Read the model definition and answer for the solid it produces. Units are mm, in the model's axes. Face numbers are marked on the shaded views. A direction names the side the tool comes from. Coordinates: 2 decimals unless noted, no trailing zeros. Write each loop counter-clockwise with the first axis right and the second up, starting at its lowest first coordinate (ties: lowest second). Pieces come first, ordered by that corner, then holes.
(1) Find the intervals of material crossed by probe 1 along X at (y, z) = (3, 22); probe 2 along X at (y, z) = (-8.5, 15.75) (3 decimals); probe 3 along Z at (x, y) = (-3, -8), in increasing order.
(2) Section D-D on z = 12.7 is taken. State how many separate pieces and enclosed holes the cut face has, then the cut area to 3 significant figures.
(3) Which of the six approach directions +Z, -Z, +X, -X, +Y, -Y give full straight-line access (tool end or side, diameter ignored) to the marked faces 4 and 5?
(4) Section A-A on x = -4 is taken. Write down the section's boundary in (y, z) (3 decimals), then the cut area to 3 significant figures.
(5) Given pin 1 (4 mm diameter, centred on x = -4.5, z = 19, fed in from +Y); pin 2 (2 mm diameter, centred on x = -1, y = 17.5, fed in from -Z); pin 3 (6 mm diameter, centred on y = -9.5, z = 9.5, fed in from +X); pin 4 (2.5 mm diameter, centred on x = 6, z = 15, fed in from +Y), each flat-ended and moving along its own axis, determine where each tip first touches the part or whether it passes through.
(6) Section B-B on y = 3 is taken. Write down the section's boundary in (x, z), then the cut area to 3 significant figures.
(7) The mould has two halves that part along Z. Classify the marked faces 1, 2 and 3: +Z half, -Z half, draft (parallel to the pull), parting line (faces both ways), or undercut.
(8) Section C-C on z = 3.75 is taken. Write down the section's boundary in (x, y) (3 decimals).
from build123d import *

# Parameters (mm, degrees)
BOSS_EXTRUDE1_DEPTH = 25.4
SKETCH2_R           = 6.35
CUT_EXTRUDE1_DEPTH  = 8.89
SKETCH3_R           = 3.175
CUT_EXTRUDE2_DEPTH  = 6.35
SKETCH4_W           = 0.635
SKETCH4_H           = 18.796
CUT_EXTRUDE3_DEPTH  = 40.162657148
SKETCH5_R           = 1.905
CUT_EXTRUDE4_DEPTH  = 40.416561089


with BuildPart() as part:
    # Sketch1 → Boss-Extrude1 (new body)
    with BuildSketch(Plane.XY):
        with BuildLine():
            ThreePointArc((-14.355971037, 17.457748951), (-15.128392597, 15.680502137), (-15.3924, 13.760725746))
            Line((-15.3924, 13.760725746), (-15.3924, 0.762))
            Line((-15.3924, 0.762), (-15.3924, -11.938))
            ThreePointArc((-15.3924, -11.938), (-13.309343428, -16.966943428), (-8.2804, -19.05))
            Line((-8.2804, -19.05), (8.2804, -19.05))
            ThreePointArc((8.2804, -19.05), (13.309343428, -16.966943428), (15.3924, -11.938))
            Line((15.3924, -11.938), (15.3924, 0.762))
            Line((15.3924, 0.762), (15.3924, 13.760725746))
            ThreePointArc((15.3924, 13.760725746), (15.128392597, 15.680502137), (14.355971037, 17.457748951))
            ThreePointArc((14.355971037, 17.457748951), (0, 25.527), (-14.355971037, 17.457748951))
        make_face()
        with BuildLine():
            Line((-9.2964, 0.762), (-9.2964, 13.760725746))
            ThreePointArc((-9.2964, 13.760725746), (-9.258684657, 14.034979516), (-9.14833872, 14.288871918))
            ThreePointArc((-9.14833872, 14.288871918), (0, 19.431), (9.14833872, 14.288871918))
            ThreePointArc((9.14833872, 14.288871918), (9.258684657, 14.034979516), (9.2964, 13.760725746))
            Line((9.2964, 13.760725746), (9.2964, 0.762))
            ThreePointArc((9.2964, 0.762), (8.99882049, 0.04357951), (8.2804, -0.254))
            Line((8.2804, -0.254), (-8.2804, -0.254))
            ThreePointArc((-8.2804, -0.254), (-8.99882049, 0.04357951), (-9.2964, 0.762))
        make_face(mode=Mode.SUBTRACT)
    extrude(amount=BOSS_EXTRUDE1_DEPTH)

    # Sketch2 → Cut-Extrude1 (cut)
    with BuildSketch(Plane(origin=(15.3924, 0, 0), x_dir=(0, 0, -1), z_dir=(1, 0, 0))):
        with Locations(Location((-12.7, -9.525, 0), (0, 0, 90))):
            Circle(SKETCH2_R)
    extrude(amount=-CUT_EXTRUDE1_DEPTH, mode=Mode.SUBTRACT)

    # Sketch3 → Cut-Extrude2 (cut)
    with BuildSketch(Plane(origin=(6.5024, 0, 0), x_dir=(0, 0, -1), z_dir=(1, 0, 0))):
        with Locations(Location((-12.7, -9.525, 0), (0, 0, 90))):
            Circle(SKETCH3_R)
    extrude(amount=-CUT_EXTRUDE2_DEPTH, mode=Mode.SUBTRACT)

    # Sketch4 → Cut-Extrude3 (cut, through all)
    with BuildSketch(Plane.XY.offset(25.4)):
        with Locations((0.3175, -9.652)):
            Rectangle(SKETCH4_W, SKETCH4_H)
        with Locations((-0.3175, -9.652)):
            Rectangle(SKETCH4_W, SKETCH4_H)
    extrude(amount=-CUT_EXTRUDE3_DEPTH, mode=Mode.SUBTRACT)

    # Sketch5 → Cut-Extrude4 (cut, through all)
    with BuildSketch(Plane(origin=(-0.635, 0, 0), x_dir=(0, 0, -1), z_dir=(1, 0, 0))):
        with Locations(Location((-12.7, -9.525, 0), (0, 0, 90))):
            Circle(SKETCH5_R)
    extrude(amount=-CUT_EXTRUDE4_DEPTH, mode=Mode.SUBTRACT)


solid = part.part
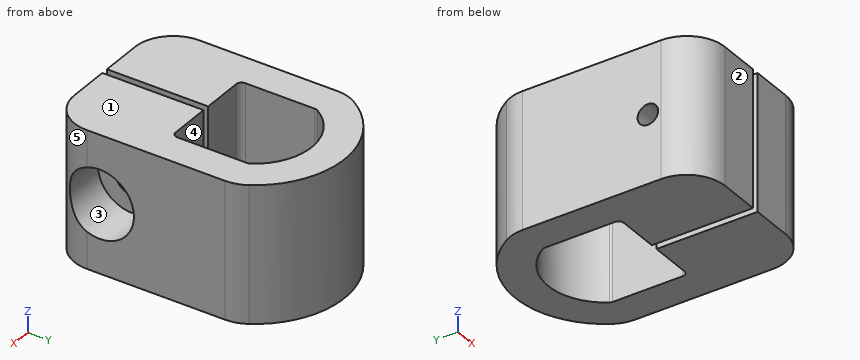
Response:
1. probe 1: x = -15.39 to -9.3, 9.3 to 15.39
1. probe 2: x = -15.392 to -0.635, 0.635 to 6.502
1. probe 3: z = 0 to 11.56, 13.84 to 25.4
2. separate pieces: 3
2. enclosed holes: 0
2. area: 698 mm2
3. face 4: +Z, -Z
3. face 5: +Z, -Z, +X, -Y
4. outline: (-19.05, 0) - (-0.254, 0) - (-0.254, 25.4) - (-19.05, 25.4) - close; (18.656, 0) - (25.044, 0) - (25.044, 25.4) - (18.656, 25.4) - close; hole circle Ø3.81 at (-9.525, 12.7)
4. area: 628 mm2
5. pin 1: stops at y = 25.34
5. pin 2: passes through
5. pin 3: stops at x = 6.5
5. pin 4: stops at y = 24.84
6. outline: (-15.39, 0) - (-9.3, 0) - (-9.3, 25.4) - (-15.39, 25.4) - close; (9.3, 0) - (15.39, 0) - (15.39, 25.4) - (9.3, 25.4) - close
6. area: 310 mm2
7. face 1: +Z half
7. face 2: draft
7. face 3: undercut
8. outline: (-15.392, -11.938) arc R7.112 ccw to (-8.28, -19.05) - (-0.635, -19.05) - (-0.635, -0.254) - (-8.28, -0.254) arc R1.016 cw to (-9.296, 0.762) - (-9.296, 13.761) arc R1.016 cw to (-9.148, 14.289) arc R10.709 cw to (9.148, 14.289) arc R1.016 cw to (9.296, 13.761) - (9.296, 0.762) arc R1.016 cw to (8.28, -0.254) - (0.635, -0.254) - (0.635, -19.05) - (8.28, -19.05) arc R7.112 ccw to (15.392, -11.938) - (15.392, 13.761) arc R7.112 ccw to (14.356, 17.458) arc R16.805 ccw to (-14.356, 17.458) arc R7.112 ccw to (-15.392, 13.761) - close
